```python
from build123d import *

# Parameters (mm, degrees)
F1_DEPTH = 40


with BuildPart() as f1:
    # F0 (on Top) → F1 (new body)
    with BuildSketch(Plane.XY):
        with BuildLine():
            ThreePointArc((-5, 49.749372), (0, 50), (5, 49.749372))
            Line((5, 49.749372), (5, 60))
            Line((5, 60), (-5, 60))
            Line((-5, 60), (-5, 49.749372))
        make_face()
        with BuildLine():
            ThreePointArc((-14, 48), (-9.540182, 49.081411), (-5, 49.749372))
            Line((-5, 49.749372), (-5, 60))
            ThreePointArc((-5, 60), (-7.5, 52.5), (-14, 48))
        make_face()
        with BuildLine():
            ThreePointArc((5, 49.749372), (9.540182, 49.081411), (14, 48))
            ThreePointArc((14, 48), (7.5, 52.5), (5, 60))
            Line((5, 60), (5, 49.749372))
        make_face()
        with BuildLine():
            ThreePointArc((40.703194, 26.929177), (40.355564, 29.001385), (39.350738, 30.846709))
            ThreePointArc((39.350738, 30.846709), (28.020245, 41.410939), (14, 48))
            ThreePointArc((14, 48), (9.540182, 49.081411), (5, 49.749372))
            Line((5, 49.749372), (-5, 49.749372))
            ThreePointArc((-5, 49.749372), (-9.540182, 49.081411), (-14, 48))
            ThreePointArc((-14, 48), (-28.020245, 41.410939), (-39.350738, 30.846709))
            ThreePointArc((-39.350738, 30.846709), (-40.355564, 29.001385), (-40.703194, 26.929177))
            Line((-40.703194, 26.929177), (-40.703194, 23.5))
            ThreePointArc((-40.703194, 23.5), (0, 47), (40.703194, 23.5))
            Line((40.703194, 23.5), (40.703194, 26.929177))
        make_face()
        with BuildLine():
            Line((-5, 49.749372), (5, 49.749372))
            ThreePointArc((5, 49.749372), (0, 50), (-5, 49.749372))
        make_face()
    extrude(amount=F1_DEPTH)


solid = f1.part
```
Can you work these out from the model? Positions are in its coordinate system, mm. Give positions to 0.01 mm unless a question says otherwise; leave off trailing zeros. Write each loop counter-clockwise with the first axis right and the second up, starting at its lowest first coordinate (ties: lowest second). Pieces come first, ordered by that corner, then holes. Notation, with made-up numbers: (-18.5, 33.25) -> (-9.5, 33.25) arc R29 cw to (-9.5, 66.25) -> close; hole circle Ø1 at (0, 58). An arc over 180 degrees is marked (long way). One line per item, written item: value.
Q1. For P1, Ø1, axis at x = 6.5, z = 7, coming from the +Y side; P2, Ø4, axis at x = -32, z = 9, coming from the +Y side; P3, Ø4, axis at y = 43, z = 31.5, coming from the +X side, each with a flat end and sliding along its axis, tell me the tip position at first contact or that it passes through.
Results found:
P1: stops at y = 55.1
P2: stops at y = 40
P3: stops at x = 28.62
Q2. Imagine slicing it at B-B on y = 34. Please give me the cut outline in (x, z), and give its area (3 significant figures).
Results found:
outline: (-36.66, 0) -> (-32.45, 0) -> (-32.45, 40) -> (-36.66, 40) -> close; (32.45, 0) -> (36.66, 0) -> (36.66, 40) -> (32.45, 40) -> close
area: 337 mm^2
Q3. Imagine slicing it at C-C on x = 35. Please give me the cut outline in (y, z), and give its area (3 significant figures).
Results found:
outline: (31.37, 0) -> (35.71, 0) -> (35.71, 40) -> (31.37, 40) -> close
area: 174 mm^2
Q4. Imagine slicing it at D-D on y = 49.5. Please give me the cut outline in (x, z), and give its area (3 significant figures).
Results found:
outline: (-10.72, 0) -> (10.72, 0) -> (10.72, 40) -> (-10.72, 40) -> close
area: 857 mm^2
Q5. Please list where these lines run through material, in increasing order: line 1 (X direction, y = 38, z = 38); line 2 (X direction, y = 32.5, z = 7.5); line 3 (Y direction, x = 26.5, z = 32). Write a range as [from, to].
Results found:
line 1: x = [-32.5, -27.66], [27.66, 32.5]
line 2: x = [-38, -33.95], [33.95, 38]
line 3: y = [38.82, 42.4]
Q6. Imagine slicing it at A-A on z = 21.5. Please give me the cut outline in (x, y).
Results found:
outline: (-40.7, 23.5) arc R47 cw to (40.7, 23.5) -> (40.7, 26.93) arc R6.35 ccw to (39.35, 30.85) arc R50 ccw to (14, 48) arc R12.5 cw to (5, 60) -> (-5, 60) arc R12.5 cw to (-14, 48) arc R50 ccw to (-39.35, 30.85) arc R6.35 ccw to (-40.7, 26.93) -> close
